Work out the finished part from the listing and answer in its coordinate system (mm). Round coordinates to 2 decimals unless told otherwise and drop trailing zeros. Order: outer loops, then holes, each group sorted by start corner. A loop starts at its lowest first (then second) coordinate and runs counter-clockwise, first axis right, second up. Notation, with made-up numbers: (-22, -13) -> (-5, -13) arc R9 ccw to (-5, -1) -> close; hole circle Ø4 at (-12, 50). An arc over 180 degrees is marked (long way). Use one line per item in the form item = value.
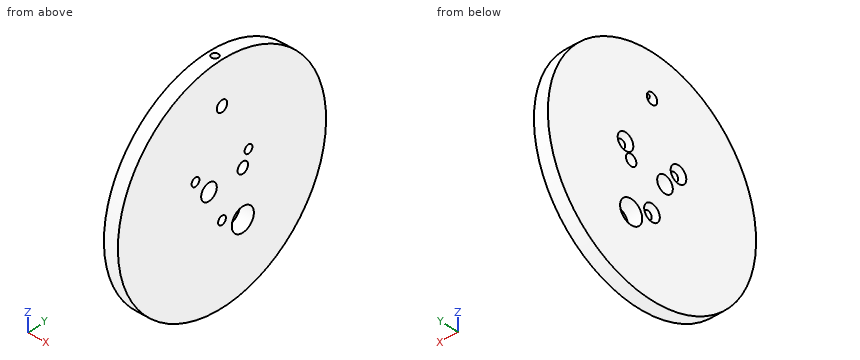
```python
from build123d import *

# Parameters (mm, degrees)
F0_W            = 5
F0_H            = 40
F3_D            = 4
F4_D            = 4
F5_D            = 6
F6_D            = 8.5
F8_D            = 3
F8_CSINK_D      = 6
F8_CSINK_ANGLE  = 90
F8_COPIES_COUNT = 3
F11_D           = 2.5
F11_DEPTH       = 14.6
F11_START       = 0.0195361
F11_TIP         = 0.7510757738


# Not quite as in the source:
# - a pattern or mirror of a feature is missing from the dataset's text; its kind, count and spacing are read off the source's solid


with BuildPart() as f1:
    # F0 (on Front) → F1 (revolve)
    with BuildSketch(Plane.XZ):
        with Locations((2.5, 20)):
            Rectangle(F0_W, F0_H)
    revolve(axis=Axis((2.5, 0, 0), (-1, 0, 0)))

    # F3 (through all)
    with Locations(Plane.YZ.offset(5)):
        with Locations((8, 1)):
            Hole(F3_D / 2)

    # F4 (through all)
    with Locations(Plane.YZ.offset(5)):
        with Locations((0, 25)):
            Hole(F4_D / 2)

    # F5 (through all)
    with Locations(Plane.YZ.offset(5)):
        with Locations((-5, 0)):
            Hole(F5_D / 2)

    # F6 (through all)
    with Locations(Plane.YZ.offset(5)):
        with Locations((8, -15.6675087226)):
            Hole(F6_D / 2)

    # F8 (through all)
    with Locations(Plane(origin=(0, 0, 0), x_dir=(0, -1, 0), z_dir=(-1, 0, 0))):
        with Locations((0, -11.75)):
            f8 = CounterSinkHole(F8_D / 2, F8_CSINK_D / 2, counter_sink_angle=F8_CSINK_ANGLE)

    # F8_copies: F8 ×3 about axis
    f8_copies_axis = Axis((0, 0, 0), (1, 0, 0))
    for i in range(1, F8_COPIES_COUNT):
        add(f8.rotate(f8_copies_axis, i * 360 / F8_COPIES_COUNT), mode=Mode.SUBTRACT)

    # F11
    # its depths count from where the whole tool has entered the part; down to there all is cleared
    with Locations(Plane.XY.offset(40).offset(-F11_START)):
        with Locations((2.5, 0)):
            Hole(F11_D / 2, depth=F11_DEPTH)
            with Locations((0, 0, -(F11_DEPTH + F11_TIP / 2))):  # 118° drill point
                Cone(0, F11_D / 2, F11_TIP, mode=Mode.SUBTRACT)


solid = f1.part
```
Item 1: The part is cut by section B-B, the plane x = 2.6. Give the number of separate pieces and of enclosed holes in the cut face, and give its area (3 significant figures).
Findings:
separate_pieces = 1
enclosed_holes = 6
area = 4,860 mm^2
Item 2: Consider line 1 along Y through (x, z) = (3.2, -11.75); line 2 along X through (y, z) = (0, 32.5); line 3 along Y through (x, z) = (1.45, 6.5). Determine where each line is inside the solid, lowest interval first.
Findings:
line_1 = -38.24 to -1.5, 1.5 to 6.35, 9.65 to 38.24
line_2 = 0 to 1.25, 3.75 to 5
line_3 = -39.47 to -11.59, -8.76 to 8.76, 11.59 to 39.47
Item 3: The part is cut by section D-D, the plane z = -26. Give the vertices of the cut face in (x, y).
Findings:
outline = (0, -30.4) -> (5, -30.4) -> (5, 30.4) -> (0, 30.4) -> close
Item 4: A flat-ended cylindrical pin translates along its axis: P1, Ø3, axis at x = 1.5, z = 7, coming from the +Y side. Find the tip coordinate at first contact, or state that the pin passes through.
Findings:
P1 = 39.62
Item 5: The part is cut by section A-A, the plane y = 0. Give the vertices of the cut face in (x, z), and give its area (3 significant figures).
Findings:
outline = (0, -40) -> (5, -40) -> (5, -13.25) -> (1.5, -13.25) -> (0, -14.75) -> close; (0, -8.75) -> (1.5, -10.25) -> (5, -10.25) -> (5, 23) -> (0, 23) -> close; (0, 27) -> (1.25, 27) -> (1.25, 40) -> (0, 40) -> close; (3.75, 27) -> (5, 27) -> (5, 40) -> (3.75, 40) -> close
area = 330 mm^2
